Read the model definition and answer for the solid it produces. Units are mm, in the model's axes. Coordinates: 2 decimals unless noted, no trailing zeros. Order: outer loops, then holes, each group sorted by start corner. A loop starts at its lowest first (then second) coordinate and runs counter-clockwise, first axis right, second up. Notation, with made-up numbers: (26, 5.25) -> (77, 5.25) arc R14 ccw to (77, 12.25) -> close; hole circle Ø5 at (39, 8.25). An arc over 180 degrees is marked (long way). Use CSV: the item, a comma, the result in double quotes.
```python
from build123d import *

# Parameters (mm, degrees)
SKETCH1_R           = 2.5
SKETCH1_R_2         = 1.25
BOSS_EXTRUDE1_DEPTH = 5


with BuildPart() as part:
    # Sketch1 → Boss-Extrude1 (new body)
    # profile 1 of 4: a face of its own
    with BuildSketch(Plane(origin=(0, 0, 0), x_dir=(1, 0, 0), z_dir=(0, 1, 0))):
        with Locations((0, -5)):
            Circle(SKETCH1_R)
        with Locations(Location((0, -5, 0), (0, 0, 270))):
            Circle(SKETCH1_R_2, mode=Mode.SUBTRACT)
    # profile 2 of 4: a face of its own
    with BuildSketch(Plane(origin=(0, 0, 0), x_dir=(1, 0, 0), z_dir=(0, 1, 0))):
        with BuildLine():
            Line((22.5, -10), (22.5, 40))
            ThreePointArc((22.5, 40), (19.579674257, 37.535588048), (17.641338984, 40.828684628))
            ThreePointArc((17.641338984, 40.828684628), (8.619996831, 18.113334742), (-2.195652157, -3.80454544))
            ThreePointArc((-2.195652157, -3.80454544), (0.616793972, -2.577281445), (2.5, -5))
            ThreePointArc((2.5, -5), (1.888934091, -6.637659305), (0.354457601, -7.474744393))
            ThreePointArc((0.354457601, -7.474744393), (9.883853248, -7.964587007), (18.522657697, -12.016794417))
            ThreePointArc((18.522657697, -12.016794417), (18.869370918, -7.770274035), (22.5, -10))
        make_face()
    # profile 3 of 4: a face of its own
    with BuildSketch(Plane(origin=(0, 0, 0), x_dir=(1, 0, 0), z_dir=(0, 1, 0))):
        with Locations((20, -10)):
            Circle(SKETCH1_R)
        with Locations(Location((20, -10, 0), (0, 0, 270))):
            Circle(SKETCH1_R_2, mode=Mode.SUBTRACT)
    # profile 4 of 4: a face of its own
    with BuildSketch(Plane(origin=(0, 0, 0), x_dir=(1, 0, 0), z_dir=(0, 1, 0))):
        with Locations((20, 40)):
            Circle(SKETCH1_R)
        with Locations(Location((20, 40, 0), (0, 0, 270))):
            Circle(SKETCH1_R_2, mode=Mode.SUBTRACT)
    extrude(amount=BOSS_EXTRUDE1_DEPTH)


solid = part.part
```
Item 1: Each of these flat-tipped pins is pushed along its axis until it touches: P1, Ø1, axis at y = 2.5, z = -15, coming from the -X side; P2, Ø10, axis at x = 2, z = -20.5, coming from the +Y side (3 decimals); P3, Ø3, axis at x = 8.5, y = 1.5, coming from the -Z side. Where does it stop, or does it pass through?
Return value:
P1,"stops at x = 6.99"
P2,"passes through"
P3,"stops at z = -21.27"
Item 2: The mould has two halves that part along X. Classify faces 1 (the cylindrical face through (21.096, 2.465, 12.247)), 2 (the cylindrical face through (0.05, 2.46, 3.75)), 3 (the flat face through (22.5, 2, -15)), 4 (the cylindrical face through (19.24, 2.46, -40.99)): +X half, -X half, draft (parallel to the pull), parting line (faces both ways), or undercut.
Return value:
face 1,"parting line"
face 2,"undercut"
face 3,"+X half"
face 4,"undercut"
Item 3: Straight lines are drawn through the part: line 1 along X through (y, z) = (3.4, 5); line 2 along X through (y, z) = (2, 4.5); line 3 along Z through (x, y) = (-0.5, 2.8). For each, find the intervals that lie inside material, in ascending order.
Return value:
line 1,"x = -2.5 to -1.25, 1.25 to 22.5"
line 2,"x = -2.45 to -1.15, 1.15 to 22.5"
line 3,"z = 0.65 to 3.85, 6.15 to 7.45"
Item 4: Find section C-C, the plane y = 3.3. Give the vertices of the cut face in (x, z), then the cut area to 3 significant figures.
Return value:
outline,"(-2.2, 3.8) arc R304.23 cw to (17.64, -40.83) arc R2.5 ccw to (22.5, -40) -> (22.5, 10) arc R2.5 ccw to (18.52, 12.02) arc R24.8 cw to (0.35, 7.47) arc R2.5 ccw to start; hole circle Ø2.5 at (0, 5); hole circle Ø2.5 at (20, -40); hole circle Ø2.5 at (20, 10)"
area,"746 mm^2"
Item 5: Find section A-A, the plane z = 5. Give the vertices of the cut face in (x, y).
Return value:
outline,"(-2.5, 0) -> (-1.25, 0) -> (-1.25, 5) -> (-2.5, 5) -> close; (1.25, 0) -> (22.5, 0) -> (22.5, 5) -> (1.25, 5) -> close"
Item 6: Find section D-D, the plane z = -2.5. Give the vertices of the cut face in (x, y).
Return value:
outline,"(1.14, 0) -> (22.5, 0) -> (22.5, 5) -> (1.14, 5) -> close"
Item 7: Find section B-B, the plane x = 20. Give the vertices of the cut face in (y, z).
Return value:
outline,"(0, -42.5) -> (5, -42.5) -> (5, -41.25) -> (0, -41.25) -> close; (0, -38.75) -> (5, -38.75) -> (5, 8.75) -> (0, 8.75) -> close; (0, 11.25) -> (5, 11.25) -> (5, 12.5) -> (0, 12.5) -> close"
